Check sheet for the modelled part. Datum: model origin and axes. Units: mm. A direction names the side the tool comes from. Give positions to 0.01 mm unless a question says otherwise; leave off trailing zeros. Order: outer loops, then holes, each group sorted by start corner. A loop starts at its lowest first (then second) coordinate and runs counter-clockwise, first axis right, second up.
Item 1: Sectioned sample at D-D on z = -29. Record the boundary of the cut face in (x, y).
Item 2: Access from +Z, -Z, +X, -X, +Y, -Y to the whole of each face (thin tool, end or side, straight path). Record for faces 1 (the cylindrical face through (-48.728, -3.451, -27.587)), 2 (the cylindrical face through (-19.24, -3.45, 11.46)).
Item 3: Release check for a two-part mould opening along Z. For faces 3 (the cylindrical face through (-0.302, -3.451, -22.393)), 4 (the cylindrical face through (19.544, -3.451, 10.935)), 5 (the cylindrical face through (-2.395, -3.451, -10.787)), 6 (the flat face through (-11, 0, 3)) record: released by +Z, released by -Z, zero draft, split by the parting line, or undercut.
Item 4: Sectioned sample at A-A on x = 0. Record the boundary of the cut face in (y, z).
Item 5: Sectioned sample at C-C on y = -3.5. Record the boundary of the cut face in (x, z).
Item 6: Material ranges on line 1 along Z through (x, y) = (0, -2.75); line 2 along Z through (x, y) = (-4, -0.5); line 3 along Z through (x, y) = (-29.5, -4), recorded low to high.
Item 7: Sectioned sample at B-B on z = -2. Record the boundary of the cut face in (x, y).
Item 8: Gauge pin test, flat ends, axial feed: P1, Ø1.5, axis at x = -36.5, y = -5, coming from the -Z side; P2, Ø1, axis at y = -3.5, z = -23.5, coming from the +X side; P3, Ø3, axis at x = -23, y = -1.5, coming from the -Z side. Record the tip position at first contact, or that the pin passes through.
from build123d import *

# Parameters (mm, degrees)
F0_R     = 11.05
F1_DEPTH = 7


with BuildPart() as f1:
    # F0 (on Front) → F1 (new body)
    with BuildSketch(Plane.XZ):
        with BuildLine():
            ThreePointArc((-18.641016, -20), (-23.243086, -8.771145), (-34.401914, -4.001787))
            ThreePointArc((-34.401914, -4.001787), (-48.497423, -28), (-20.666606, -27.792039))
            ThreePointArc((-20.666606, -27.792039), (-19.155691, -24.025509), (-18.641016, -20))
        make_face()
        with Locations((-34.641016, -20)):
            Circle(F0_R, mode=Mode.SUBTRACT)
        with BuildLine():
            ThreePointArc((13.735308, 31.793825), (0, 24), (-13.735308, 31.793825))
            ThreePointArc((-13.735308, 31.793825), (-19.391728, 11.195819), (-34.401914, -4.001787))
            ThreePointArc((-34.401914, -4.001787), (-23.243086, -8.771145), (-18.641016, -20))
            ThreePointArc((-18.641016, -20), (-19.155691, -24.025509), (-20.666606, -27.792039))
            ThreePointArc((-20.666606, -27.792039), (0, -22.391639), (20.666606, -27.792039))
            ThreePointArc((20.666606, -27.792039), (20.78461, -12), (34.401914, -4.001787))
            ThreePointArc((34.401914, -4.001787), (19.391728, 11.195819), (13.735308, 31.793825))
        make_face()
        Circle(F0_R, mode=Mode.SUBTRACT)
        with BuildLine():
            ThreePointArc((13.735308, 31.793825), (15.423439, 35.74353), (16, 40))
            ThreePointArc((16, 40), (-4.25647, 55.423439), (-13.735308, 31.793825))
            ThreePointArc((-13.735308, 31.793825), (0, 24), (13.735308, 31.793825))
        make_face()
        with Locations((0, 40)):
            Circle(F0_R, mode=Mode.SUBTRACT)
        with BuildLine():
            ThreePointArc((50.641016, -20), (45.869871, -8.60207), (34.401914, -4.001787))
            ThreePointArc((34.401914, -4.001787), (20.78461, -12), (20.666606, -27.792039))
            ThreePointArc((20.666606, -27.792039), (38.666525, -35.485325), (50.641016, -20))
        make_face()
        with Locations((34.641016, -20)):
            Circle(F0_R, mode=Mode.SUBTRACT)
    extrude(amount=F1_DEPTH)


solid = f1.part
Report:
1. outline: (-47.87, -7) - (-41.05, -7) - (-41.05, 0) - (-47.87, 0) - close; (-28.23, -7) - (-21.41, -7) - (-21.41, 0) - (-28.23, 0) - close; (21.41, -7) - (28.23, -7) - (28.23, 0) - (21.41, 0) - close; (41.05, -7) - (47.87, -7) - (47.87, 0) - (41.05, 0) - close
2. face 1: +Y, -Y
2. face 2: -X, +Y, -Y
3. face 3: released by -Z
3. face 4: undercut
3. face 5: undercut
3. face 6: zero draft
4. outline: (-7, -22.39) - (0, -22.39) - (0, -11.05) - (-7, -11.05) - close; (-7, 11.05) - (0, 11.05) - (0, 28.95) - (-7, 28.95) - close; (-7, 51.05) - (0, 51.05) - (0, 56) - (-7, 56) - close
5. outline: (-34.4, -4) arc R16 ccw (long way) to (-20.67, -27.79) arc R42.24 cw to (20.67, -27.79) arc R16 ccw (long way) to (34.4, -4) arc R42.24 cw to (13.74, 31.79) arc R16 ccw to (16, 40) arc R16 ccw (long way) to (-13.74, 31.79) arc R42.24 cw to start; hole circle Ø22.1 at (-34.64, -20); hole circle Ø22.1 at (0, 0); hole circle Ø22.1 at (0, 40); hole circle Ø22.1 at (34.64, -20)
6. line 1: z = -22.39 to -11.05, 11.05 to 28.95, 51.05 to 56
6. line 2: z = -22.58 to -10.3, 10.3 to 29.7, 50.3 to 55.49
6. line 3: z = -35.15 to -29.78, -10.22 to -0.6
7. outline: (-31.34, -7) - (-10.87, -7) - (-10.87, 0) - (-31.34, 0) - close; (10.87, -7) - (31.34, -7) - (31.34, 0) - (10.87, 0) - close
8. P1: stops at z = -35.96
8. P2: stops at x = 50.36
8. P3: stops at z = -32.38
